For this review, take the finished solid that the model builds, in its own axes (mm). A direction names the side the tool comes from. Coordinates: 2 decimals unless noted, no trailing zeros. Loops run counter-clockwise (first coordinate to the right, second up) from the corner with the lowest first, then second, coordinate; pieces in that order, holes last. Notation, with made-up numbers: (6.5, 4) - (12.5, 4) arc R13 cw to (12.5, 17) - close; hole circle Ø2 at (-26.75, -28). An arc over 180 degrees is marked (long way). Answer as a JSON object with one key per item and string values. Group by question number.
Item 1: Tool access review of faces 1 (the flat face through (6, 1.3, -10)), 2 (the flat face through (4.95, 1, -10)), 3 (the flat face through (15.3, 1, -18)), 4 (the flat face through (6, 1, -10.9)): name each direction out of +Z, -Z, +X, -X, +Y, -Y from which nothing blocks a thin tool from reaching the whole face with its end or side.
Item 2: To check wall thickness, follow line 1 (X direction, y = -1.1, z = -1.54); line 2 (X direction, y = -0.85, z = -28); line 3 (Z direction, x = 13.25, y = 1.9). State the ranges of each line that lie inside material, in increasing order.
Item 3: We need section B-B (x = 9). Give the boundary of the cut face in (y, z), then the cut area to 3 significant figures.
Item 4: We need section C-C (z = -15.54). Give the boundary of the cut face in (x, y), then the cut area to 3 significant figures.
Item 5: Clearance check with flat-ended pins moving along their axes: pin 1 (10 mm diameter, centred on x = 12, z = -13, fed in from +Y); pin 2 (1.3 mm diameter, centred on x = 9, z = -28, fed in from -Y); pin 3 (0.6 mm diameter, centred on x = 6, z = -10.5, fed in from +Y); pin 4 (3 mm diameter, centred on x = 12.5, y = 2, fed in from +Z). State where each tip first meets the part, or that it passes through.
Item 6: We need section A-A (y = 0.8). Give the boundary of the cut face in (x, z).
Item 7: Mouldability with a two-part tool opening along X and no side actions: class faces 5 (the flat face through (2.7, 1, -18)), 6 (the flat face through (9, 3, -19)), 7 (the flat face through (9, 1, -24.84)) as released by +X, released by -X, zero draft, split by the parting line, or undercut.
Item 8: We need section D-D (x = 12). Give the boundary of the cut face in (y, z).
from build123d import *

# Parameters (mm, degrees)
SKETCH1_W           = 12.6
SKETCH1_H           = 12.6
BOSS_EXTRUDE1_DEPTH = 1.3
SKETCH3_R           = 1.29375
BOSS_EXTRUDE3_DEPTH = 2.7
DRAFT1_ANGLE        = 26
SKETCH4_W           = 12.6
SKETCH4_H           = 12.6
BOSS_EXTRUDE4_DEPTH = 1.7
SKETCH5_W           = 17.8
SKETCH5_H           = 30.8
BOSS_EXTRUDE5_DEPTH = 1.6
FILLET1_SIZE        = 0.7
SKETCH7_R           = 1.1
CUT_EXTRUDE1_DEPTH  = 36.933549783
SKETCH8_W           = 2.7
SKETCH8_H           = 1.2
CAPACITOR_DEPTH     = 1.3
FILLET5_R           = 0.7


with BuildPart() as part:
    # Sketch1 → Boss-Extrude1 (new body)
    with BuildSketch(Plane(origin=(0, 0, 0), x_dir=(1, 0, 0), z_dir=(0, 1, 0))):
        with Locations((9, 18.54)):
            Rectangle(SKETCH1_W, SKETCH1_H)
    extrude(amount=BOSS_EXTRUDE1_DEPTH)

    # Sketch3 → Boss-Extrude3 (add)
    with BuildSketch(Plane(origin=(0, 1.3, 0), x_dir=(1, 0, 0), z_dir=(0, 1, 0))):
        with Locations(Location((6, 21.54, 0), (0, 0, 90))):
            Circle(SKETCH3_R)
        with Locations(Location((12, 21.54, 0), (0, 0, 90))):
            Circle(SKETCH3_R)
        with Locations(Location((12, 15.54, 0), (0, 0, 90))):
            Circle(SKETCH3_R)
        with Locations(Location((6, 15.54, 0), (0, 0, 90))):
            Circle(SKETCH3_R)
    extrude(amount=BOSS_EXTRUDE3_DEPTH)

    # Draft1
    draft1_faces = [part.faces().sort_by_distance(p)[0] for p in [
        (6, 2.65, -14.24625),
        (12, 2.65, -14.24625),
        (12, 2.65, -20.24625),
        (6, 2.65, -20.24625),
    ]]
    draft(draft1_faces, Plane(origin=(6, 4, -21.54), x_dir=(0, 0, 1), z_dir=(0, 1, 0)), DRAFT1_ANGLE)

    # Sketch4 → Boss-Extrude4 (add)
    with BuildSketch(Plane(origin=(0, 1.3, 0), x_dir=(1, 0, 0), z_dir=(0, 1, 0))):
        with Locations((9, 18.54)):
            Rectangle(SKETCH4_W, SKETCH4_H)
    extrude(amount=BOSS_EXTRUDE4_DEPTH)

    # Sketch5 → Boss-Extrude5 (add)
    with BuildSketch(Plane.XZ):
        with Locations((9, -15.5)):
            Rectangle(SKETCH5_W, SKETCH5_H)
    extrude(amount=BOSS_EXTRUDE5_DEPTH)

    # Fillet1
    fillet1_edges = [part.edges().sort_by_distance(p)[0] for p in [
        (2.7, 3, -18.54),
        (9, 3, -12.24),
        (15.3, 3, -18.54),
        (9, 3, -24.84),
    ]]
    chamfer(fillet1_edges, length=FILLET1_SIZE)

    # Sketch7 → Cut-Extrude1 (cut, through all)
    with BuildSketch(Plane(origin=(0, 0, 0), x_dir=(1, 0, 0), z_dir=(0, 1, 0))):
        with Locations(Location((1.5, 1.54, 0), (0, 0, 270))):
            Circle(SKETCH7_R)
        with Locations(Location((9, 28, 0), (0, 0, 270))):
            Circle(SKETCH7_R)
        with Locations(Location((16.5, 1.54, 0), (0, 0, 270))):
            Circle(SKETCH7_R)
    extrude(amount=-CUT_EXTRUDE1_DEPTH, mode=Mode.SUBTRACT)

    # Sketch8 → capacitor (add)
    with BuildSketch(Plane(origin=(0, 0, 0), x_dir=(1, 0, 0), z_dir=(0, 1, 0))):
        with Locations((6.3, 10.3)):
            Rectangle(SKETCH8_W, SKETCH8_H)
    extrude(amount=CAPACITOR_DEPTH)

    # Fillet5
    fillet5_edges = [part.edges().sort_by_distance(p)[0] for p in [
        (3.4, 3, -18.54),
        (9, 3, -24.14),
        (14.6, 3, -18.54),
        (9, 3, -12.94),
        (9, 2.3, -12.24),
        (15.3, 2.3, -18.54),
        (9, 2.3, -24.84),
        (2.7, 2.3, -18.54),
    ]]
    fillet(fillet5_edges, radius=FILLET5_R)


solid = part.part
Check sheet entries:
{
 "1": {"face 1": "+Z, +X, -X, +Y", "face 2": "+Z, -X, +Y", "face 3": "+Z, -Z, +X, +Y", "face 4": "+X, -X, +Y"},
 "2": {"line 1": "x = 0.1 to 0.4, 2.6 to 15.4, 17.6 to 17.9", "line 2": "x = 0.1 to 7.9, 10.1 to 17.9", "line 3": "z = -24.84 to -12.24"},
 "3": {"outline": "(-1.6, -30.9) - (0, -30.9) - (0, -29.1) - (-1.6, -29.1) - close; (-1.6, -26.9) - (0, -26.9) - (0, -24.84) - (2.01, -24.84) arc R0.7 ccw to (2.51, -24.63) - (2.79, -24.35) arc R0.7 ccw to (3, -23.85) - (3, -13.23) arc R0.7 ccw to (2.79, -12.73) - (2.51, -12.45) arc R0.7 ccw to (2.01, -12.24) - (0, -12.24) - (0, -0.1) - (-1.6, -0.1) - close", "area": "83.0 mm2"},
 "4": {"outline": "(0.1, -1.6) - (17.9, -1.6) - (17.9, 0) - (15.3, 0) - (15.3, 2.01) arc R0.7 ccw to (15.09, 2.51) - (14.81, 2.79) arc R0.7 ccw to (14.31, 3) - (13.78, 3) - (13.29, 4) - (10.71, 4) - (10.22, 3) - (7.78, 3) - (7.29, 4) - (4.71, 4) - (4.22, 3) - (3.69, 3) arc R0.7 ccw to (3.19, 2.79) - (2.91, 2.51) arc R0.7 ccw to (2.7, 2.01) - (2.7, 0) - (0.1, 0) - close", "area": "71.9 mm2"},
 "5": {"pin 1": "stops at y = 4", "pin 2": "passes through", "pin 3": "stops at y = 1.3", "pin 4": "stops at z = -12.24"},
 "6": {"outline": "(2.7, -24.84) - (15.3, -24.84) - (15.3, -12.24) - (2.7, -12.24) - close; (4.95, -10.9) - (7.65, -10.9) - (7.65, -9.7) - (4.95, -9.7) - close"},
 "7": {"face 5": "released by -X", "face 6": "undercut", "face 7": "zero draft"},
 "8": {"outline": "(-1.6, -30.9) - (0, -30.9) - (0, -24.84) - (2.01, -24.84) arc R0.7 ccw to (2.51, -24.63) - (2.79, -24.35) arc R0.7 ccw to (3, -23.85) - (3, -23.32) - (4, -22.83) - (4, -20.25) - (3, -19.76) - (3, -17.32) - (4, -16.83) - (4, -14.25) - (3, -13.76) - (3, -13.23) arc R0.7 ccw to (2.79, -12.73) - (2.51, -12.45) arc R0.7 ccw to (2.01, -12.24) - (0, -12.24) - (0, -0.1) - (-1.6, -0.1) - close"}
}
